Part model, mm, in its own coordinate system. Face numbers are marked on the shaded views. A direction names the side the tool comes from. Round coordinates to 2 decimals unless told otherwise and drop trailing zeros. Write each loop counter-clockwise with the first axis right and the second up, starting at its lowest first coordinate (ties: lowest second). Pieces come first, ordered by that corner, then holes. Notation, with made-up numbers: (-36.75, 27) -> (13.25, 27) arc R19 ccw to (13.25, 41) -> close; hole circle Ø4 at (48, 71). An arc over 180 degrees is marked (long way). Use CSV: the item, a comma, the result in double quotes. Start each with the question number.
(1) Drop flat-ended pins along their axis: pin 1 (5 mm diameter, centred on y = 3.5, z = 5.5, fed in from -X); pin 2 (3 mm diameter, centred on x = 18, z = 26.5, fed in from +Y); pin 3 (3 mm diameter, centred on x = -19.4, z = 7.5, fed in from +Y); pin 4 (1 mm diameter, centred on y = 5, z = 11.5, fed in from +X). Give the stop position or say it passes through.
(2) Saw through at A-A (y = 0.85). Give the cut face in (x, z), plus the area to 3 significant figures.
(3) Two-plate mould, pull along Y, no slides. Class the marked faces 1, 2, 3 and 4: released by +Y, released by -Y, zero draft, split by the parting line, or undercut.
(4) Saw through at B-B (x = -2). Give the cut face in (y, z), plus the area to 3 significant figures.
(5) Saw through at C-C (z = 15). Give the cut face in (x, y).
(6) Saw through at D-D (z = 3). Give the cut face in (x, y), plus the area to 3 significant figures.
(7) Probe line 1 (X direction, y = -5.55, z = 22.5); line 2 (Z direction, x = 19.4, y = -6.5); line 3 (Y direction, x = -3, z = 26.5). List the from-to ranges inside material, lowest first. Write a range as [from, to].
(8) Which spindle directions (+Z, -Z, +X, -X, +Y, -Y) get a long thin tool onto all of the face, cutting with end or side? Do the marked faces 5 and 6. Say none if no direction does.
Autodesk Inventor part; units mm, degrees
ref_plane "YZ Plane" through (0, 0, 0) normal (1, 0, 0) x (0, 1, 0)
ref_plane "XZ Plane" through (0, 0, 0) normal (0, 1, 0) x (-1, 0, 0)
ref_plane "XY Plane" through (0, 0, 0) normal (0, 0, 1) x (1, 0, 0)
sketch "Sketch1" plane through (0, 0, 0) normal (0, 0, 1) x (1, 0, 0)
  line L0 (-10.2, -5.2) -> (10.2, -5.2)
  line L1 (10.2, -5.2) -> (10.2, 5.2)
  line L2 (10.2, 5.2) -> (-10.2, 5.2)
  line L3 (-10.2, 5.2) -> (-10.2, -5.2)
  line L4 (-10.2, -5.2) -> (10.2, 5.2) construction
  line L5 (10.2, -5.2) -> (-10.2, 5.2) construction
  line L6 (-11.9, 6.9) -> (11.9, 6.9)
  line L7 (11.9, 6.9) -> (11.9, -6.9)
  line L8 (11.9, -6.9) -> (-11.9, -6.9)
  line L9 (-11.9, -6.9) -> (-11.9, 6.9)
  point P0 (0, 0)
  dimension "d0" = 20.4
  dimension "d1" = 10.4
  dimension "d2" = 1.7
extrude "Extrusion1" add sketch "Sketch1" along normal blind 30
sketch "Sketch2" plane through (-11.9, -6.9, 0) normal (0, -1, 0) x (1, 0, 0)
  line L0 (-15, 0) -> (38.8, 0)
  line L1 (38.8, 0) -> (38.8, 30)
  line L2 (38.8, 30) -> (-15, 30)
  line L3 (-15, 30) -> (-15, 0)
  line L4 (-15, 0) -> (38.8, 30) construction
  line L5 (38.8, 0) -> (-15, 30) construction
  point P0 (11.9, 0)
  point P1 (11.9, 15)
  dimension "d5" = 53.8
  dimension "d23" = 30
extrude "Extrusion2" add sketch "Sketch2" against normal blind 1.7
sketch "Sketch3" plane through (-11.9, -5.2, 0) normal (0, 1, 0) x (1, 0, 0)
  line L0 (-15, 0) -> (38.8, 0) construction
  line L1 (0, 0) -> (0, -30) construction
  line L2 (-15, 0) -> (0, 0) construction
  line L3 (0, 0) -> (0, -15) construction
  line L4 (0, -15) -> (-15, -15) construction
  line L5 (-15, -15) -> (-15, 0) construction
  line L6 (-15, 0) -> (0, -15) construction
  line L7 (-15, 0) -> (-15, -30) construction
  line L8 (0, -15) -> (-15, -30) construction
  point P0 (11.9, 0)
  point P1 (-7.5, -7.5)
  point P2 (-7.5, -22.5)
  point P3 (-15, -7.5)
  point P4 (-7.5, 0)
  dimension "d24" = 7.5
  dimension "d25" = 7.5
hole "Hole1" at (-19.4, -5.2, 7.5) at (-19.4, -5.2, 22.5) direction (0, -1, 0) diameter 3.4 depth 5 tip angle 118
mirror "Mirror1" about plane through (0, 0, 0) normal (1, 0, 0) of "Hole1"
fillet "Fillet1" radius 7 4 edges at (26.9, -6.05, 30) (26.9, -6.05, 0) (-26.9, -6.05, 0) (-26.9, -6.05, 30)
sketch "Sketch4" plane through (11.9, 6.9, 30) normal (1, 0, 0) x (0, 0, -1)
  line L0 (30, 0) -> (0, 0) construction
  line L1 (30, -12.1) -> (0, -12.1) construction
  line L2 (0, 0) -> (30, -12.1) construction
  circle A0 centre (15, -6.05) radius 1.5
  circle A1 centre (15, -6.05) radius 2.25
  point P0 (30, -6.9)
  dimension "d16" = 3
  dimension "d17" = 0.75
extrude "Extrusion3" add sketch "Sketch4" along normal blind 2
fillet "Fillet2" radius 1 1 edges at (11.9, 0.85, 17.25)
extrude "Extrusion4" cut sketch "Sketch4" against normal blind 2 contours A0
properties part number "BeamHoldertoBack" material "ABS Plastic"
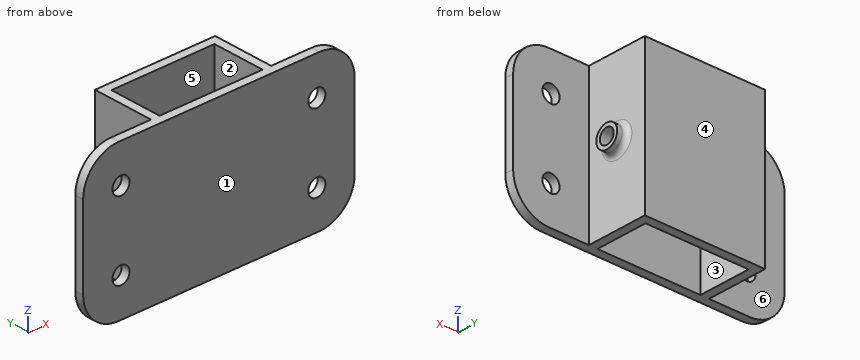
Answers:
1,pin 1,"stops at x = -11.9"
1,pin 2,"stops at y = -5.2"
1,pin 3,"passes through"
1,pin 4,"stops at x = 11.9"
2,outline,"(-11.9, 0) -> (-10.2, 0) -> (-10.2, 30) -> (-11.9, 30) -> close; (10.2, 0) -> (11.9, 0) -> (11.9, 11.75) arc R1 cw to (12.9, 12.75) -> (13.9, 12.75) -> (13.9, 13.5) -> (10.2, 13.5) -> close; (10.2, 16.5) -> (13.9, 16.5) -> (13.9, 17.25) -> (12.9, 17.25) arc R1 cw to (11.9, 18.25) -> (11.9, 30) -> (10.2, 30) -> close"
2,area,"100 mm²"
3,face 1,"released by -Y"
3,face 2,"undercut"
3,face 3,"undercut"
3,face 4,"released by +Y"
4,outline,"(-6.9, 0) -> (-5.2, 0) -> (-5.2, 30) -> (-6.9, 30) -> close; (5.2, 0) -> (6.9, 0) -> (6.9, 30) -> (5.2, 30) -> close"
4,area,"102 mm²"
5,outline,"(-26.9, -6.9) -> (26.9, -6.9) -> (26.9, -5.2) -> (11.9, -5.2) -> (11.9, -2.4) arc R1 cw to (12.9, -1.4) -> (13.9, -1.4) -> (13.9, -0.65) -> (10.2, -0.65) -> (10.2, -5.2) -> (-10.2, -5.2) -> (-10.2, 5.2) -> (10.2, 5.2) -> (10.2, 2.35) -> (13.9, 2.35) -> (13.9, 3.1) -> (12.9, 3.1) arc R1 cw to (11.9, 4.1) -> (11.9, 6.9) -> (-11.9, 6.9) -> (-11.9, -5.2) -> (-26.9, -5.2) -> close"
6,outline,"(-25.64, -6.9) -> (25.64, -6.9) -> (25.64, -5.2) -> (11.9, -5.2) -> (11.9, 6.9) -> (-11.9, 6.9) -> (-11.9, -5.2) -> (-25.64, -5.2) -> close; hole (-10.2, -5.2) -> (10.2, -5.2) -> (10.2, 5.2) -> (-10.2, 5.2) -> close"
6,area,"163 mm²"
7,line 1,"x = [-26.9, -21.1], [-17.7, 17.7], [21.1, 26.9]"
7,line 2,"z = [0, 5.8], [9.2, 20.8], [24.2, 30]"
7,line 3,"y = [-6.9, -5.2], [5.2, 6.9]"
8,face 5,"+Z, -Z"
8,face 6,"+Z, -Z, -X, +Y"
